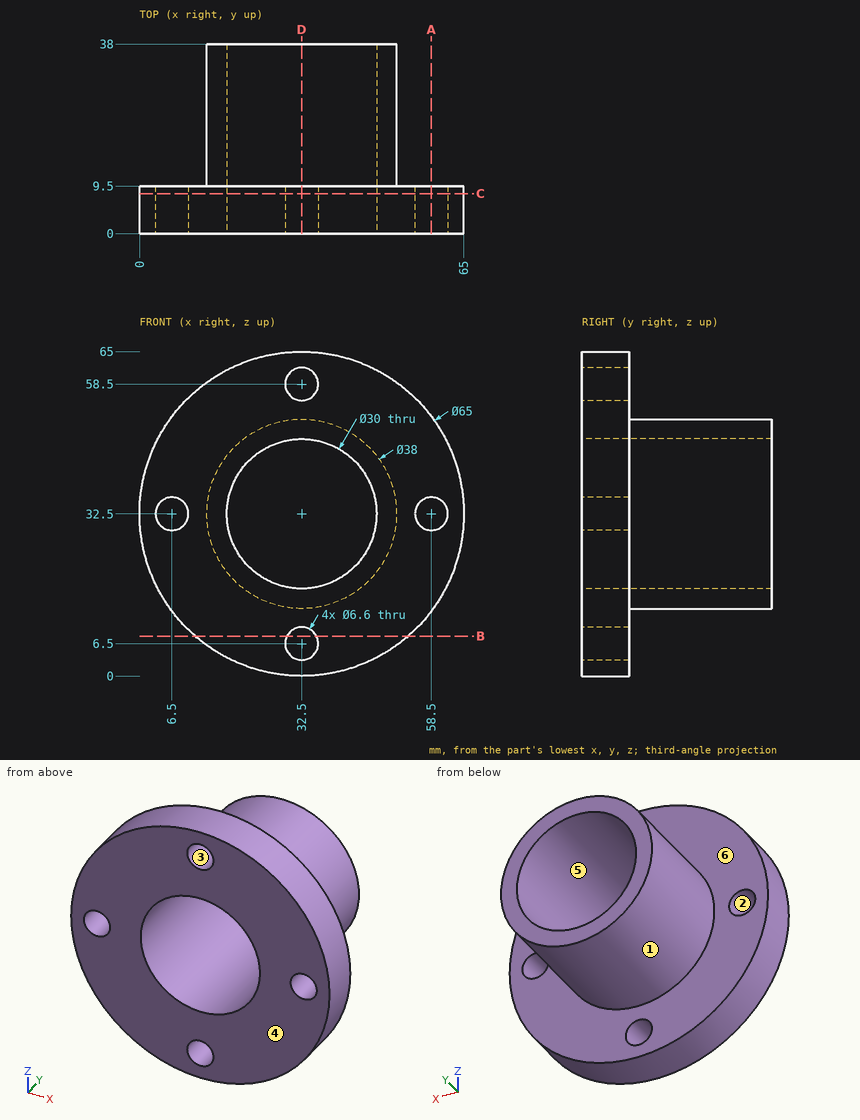
Input: dimensioned drawing with shaded views. Units: mm. Origin: part minimum x, y, z. A direction names the side the tool comes from. Coordinates: 2 decimals unless noted, no trailing zeros. Order: outer loops, then holes, each group sorted by start corner. A loop starts at its lowest first (then second) coordinate and runs counter-clockwise, first axis right, second up. Notation, with made-up numbers: M 41,15.5 L 83,15.5 A10 cw 83,21.5 Z; hole C 42.5,-5 d6. An arc over 180 degrees is marked long. Write each question's results on one line, items separated by ' | '. Start each with the question number.
Item 1: First-contact query: pin 1 Ø7.5 at (x, z) = (6.5, 32.5) entering from +Y; pin 2 Ø8 at (x, y) = (41, 6.5) entering from +Z; pin 3 Ø5.5 at (x, z) = (32.5, 58.5) entering from -Y; pin 4 Ø10 at (y, z) = (25.5, 39) entering from +X. Flat tips, straight axial feed; report the tip coordinate or a pass-through.
Item 2: Line query: probe 1 along X at (y, z) = (7.75, 32.5); probe 2 along X at (y, z) = (28.5, 32.5); probe 3 along Z at (x, y) = (32, 11.5). Output: solid intervals per line, ascending.
Item 3: Draft query along Z for the marked faces 1, 2, 3 and 4. Return one class per face: pulls with the +Z half, pulls with the -Z half, needs draft (parallel to the pull), parting line crosses it, or undercut.
Item 4: Cut plane A-A (x = 58.5). Return loops of the section in (y, z).
Item 5: Set-up query: the marked faces 5 and 6. Return all of +Z, -Z, +X, -X, +Y, -Y with unobstructed straight access to the full face (end or side cutting, diameter ignored); none if empty.
Item 6: Cut plane C-C (y = 8). Return loops of the section in (x, z), and give its area (3 significant figures).
Item 7: Cut plane D-D (x = 32.5). Return loops of the section in (y, z), and give its area (3 significant figures).
Item 8: Cut plane B-B (z = 8). Return loops of the section in (x, y), and give its area (3 significant figures).
Checked values:
1) pin 1: stops at y = 9.5 | pin 2: stops at z = 64.69 | pin 3: passes through | pin 4: stops at x = 51.44
2) probe 1: x = 0 to 3.2, 9.8 to 17.5, 47.5 to 55.2, 61.8 to 65 | probe 2: x = 13.5 to 17.5, 47.5 to 51.5 | probe 3: z = 13.51 to 17.51, 47.49 to 51.49
3) face 1: parting line crosses it | face 2: undercut | face 3: undercut | face 4: needs draft
4) outline: M 0,13 L 9.5,13 L 9.5,29.2 L 0,29.2 Z; M 0,35.8 L 9.5,35.8 L 9.5,52 L 0,52 Z
5) face 5: +Y, -Y | face 6: +Y
6) outline: C 32.5,32.5 d65; hole C 6.5,32.5 d6.6; hole C 32.5,32.5 d30; hole C 32.5,6.5 d6.6; hole C 32.5,58.5 d6.6; hole C 58.5,32.5 d6.6 | area: 2,470 mm2
7) outline: M 0,0 L 9.5,0 L 9.5,3.2 L 0,3.2 Z; M 0,9.8 L 9.5,9.8 L 9.5,13.5 L 38,13.5 L 38,17.5 L 0,17.5 Z; M 0,47.5 L 38,47.5 L 38,51.5 L 9.5,51.5 L 9.5,55.2 L 0,55.2 Z; M 0,61.8 L 9.5,61.8 L 9.5,65 L 0,65 Z | area: 435 mm2
8) outline: M 11.15,0 L 29.56,0 L 29.56,9.5 L 11.15,9.5 Z; M 35.44,0 L 53.85,0 L 53.85,9.5 L 35.44,9.5 Z | area: 350 mm2
